from build123d import *

# Parameters (mm, degrees)
SKETCH1_W                      = 347.1920001
SKETCH1_H                      = 182.714000078
BASE_FLANGE1_DEPTH             = 2.286
EDGE_FLANGE1_STRIP_W           = 10.7696
EDGE_FLANGE1_STRIP_H           = 2.286
EDGE_FLANGE1_STRIP_CUT_DEPTH   = 182.714000078
EDGE_FLANGE1_STRIP_2_W         = 10.7696
EDGE_FLANGE1_STRIP_2_H         = 2.286
EDGE_FLANGE1_STRIP_CUT_2_DEPTH = 182.714000078
EDGE_FLANGE1_DEPTH             = 182.714000078
EDGE_FLANGE1_BEND_DEPTH        = 182.714000078
EDGE_FLANGE2_STRIP_W           = 10.7696
EDGE_FLANGE2_STRIP_H           = 2.286
EDGE_FLANGE2_STRIP_CUT_DEPTH   = 345.5664001
EDGE_FLANGE2_DEPTH             = 345.5664001
SKETCH17_W                     = 40
SKETCH17_H                     = 31.75
CUT_EXTRUDE1_DEPTH             = 201.869732409
FILLET1_R                      = 2.54
F_1_8_0_1250_DOWEL_HOLE1_D     = 3.175
F_1_8_0_1250_DOWEL_HOLE1_DEPTH = 351.7640001
F_1_8_0_1250_DOWEL_HOLE1_TIP   = 0.953866233


# Sheet-metal steps are written as plain solids
with BuildPart() as part:
    # Sketch1 → Base-Flange1 (new body)
    with BuildSketch(Plane.XY):
        Rectangle(SKETCH1_W, SKETCH1_H)
    extrude(amount=-BASE_FLANGE1_DEPTH)

    # Edge-Flange1 strip (across the edge) → Edge-Flange1 strip cut (cut)
    with BuildSketch(Plane(origin=(173.59600005, 91.357000039, -2.286), x_dir=(-1, 0, 0), z_dir=(0, -1, 0))):
        with Locations((-4.572, -1.143)):
            Rectangle(EDGE_FLANGE1_STRIP_W, EDGE_FLANGE1_STRIP_H)
    extrude(amount=EDGE_FLANGE1_STRIP_CUT_DEPTH, mode=Mode.SUBTRACT)

    # Edge-Flange1 strip 2 (across the edge) → Edge-Flange1 strip cut 2 (cut)
    with BuildSketch(Plane(origin=(-173.59600005, -91.357000039, -2.286), x_dir=(1, 0, 0), z_dir=(0, 1, 0))):
        with Locations((-4.572, -1.143)):
            Rectangle(EDGE_FLANGE1_STRIP_2_W, EDGE_FLANGE1_STRIP_2_H)
    extrude(amount=EDGE_FLANGE1_STRIP_CUT_2_DEPTH, mode=Mode.SUBTRACT)

    # Edge-Flange1 section (across the edge) → Edge-Flange1 (add)
    with BuildSketch(Plane(origin=(173.59600005, 91.357000039, -2.286), x_dir=(-1, 0, 0), z_dir=(0, -1, 0))):
        with BuildLine():
            Line((-2.286, 0.8128), (-2.286, 25.4))
            Line((-2.286, 25.4), (0, 25.4))
            Line((0, 25.4), (0, 0.8128))
            ThreePointArc((0, 0.8128), (0.238063608, 0.238063608), (0.8128, 0))
            Line((0.8128, 0), (0.8128, -2.286))
            ThreePointArc((0.8128, -2.286), (-1.378382494, -1.378382494), (-2.286, 0.8128))
        make_face()
    extrude(amount=EDGE_FLANGE1_DEPTH)

    # Edge-Flange1 section 2 (across the edge) → Edge-Flange1 bend (add)
    with BuildSketch(Plane(origin=(-173.59600005, -91.357000039, -2.286), x_dir=(1, 0, 0), z_dir=(0, 1, 0))):
        with BuildLine():
            Line((-2.286, 0.8128), (-2.286, 25.4))
            Line((-2.286, 25.4), (0, 25.4))
            Line((0, 25.4), (0, 0.8128))
            ThreePointArc((0, 0.8128), (0.238063608, 0.238063608), (0.8128, 0))
            Line((0.8128, 0), (0.8128, -2.286))
            ThreePointArc((0.8128, -2.286), (-1.378382494, -1.378382494), (-2.286, 0.8128))
        make_face()
    extrude(amount=EDGE_FLANGE1_BEND_DEPTH)

    # Edge-Flange2 strip (across the edge) → Edge-Flange2 strip cut (cut)
    with BuildSketch(Plane(origin=(172.78320005, -91.357000039, -2.286), x_dir=(0, 1, 0), z_dir=(-1, 0, 0))):
        with Locations((-4.572, -1.143)):
            Rectangle(EDGE_FLANGE2_STRIP_W, EDGE_FLANGE2_STRIP_H)
    extrude(amount=EDGE_FLANGE2_STRIP_CUT_DEPTH, mode=Mode.SUBTRACT)

    # Edge-Flange2 section (across the edge) → Edge-Flange2 (add)
    with BuildSketch(Plane(origin=(172.78320005, -91.357000039, -2.286), x_dir=(0, 1, 0), z_dir=(-1, 0, 0))):
        with BuildLine():
            Line((-2.286, 0.8128), (-2.286, 19.05))
            Line((-2.286, 19.05), (0, 19.05))
            Line((0, 19.05), (0, 0.8128))
            ThreePointArc((0, 0.8128), (0.238063608, 0.238063608), (0.8128, 0))
            Line((0.8128, 0), (0.8128, -2.286))
            ThreePointArc((0.8128, -2.286), (-1.378382494, -1.378382494), (-2.286, 0.8128))
        make_face()
    extrude(amount=EDGE_FLANGE2_DEPTH)

    # Sketch17 → Cut-Extrude1 (cut, through all)
    with BuildSketch(Plane(origin=(0, 0, -2.286), x_dir=(-1, 0, 0), z_dir=(0, 0, -1))):
        with Locations((152.78320005, 75.482000039)):
            Rectangle(SKETCH17_W, SKETCH17_H)
    extrude(amount=-CUT_EXTRUDE1_DEPTH, mode=Mode.SUBTRACT)

    # Fillet1
    fillet1_edges = [part.edges().sort_by_distance(p)[0] for p in [
        (172.78320005, -92.500000039, -21.336),
        (-172.78320005, -92.500000039, -21.336),
        (-172.78320005, 59.607000039, -1.143),
        (-132.78320005, 59.607000039, -1.143),
        (-132.78320005, 91.357000039, -1.143),
        (174.73900005, 91.357000039, -27.686),
        (174.73900005, -91.357000039, -27.686),
        (-174.73900005, -91.357000039, -27.686),
        (-174.73900005, 91.357000039, -27.686),
    ]]
    fillet(fillet1_edges, radius=FILLET1_R)

    # 1/8 (0.1250) Dowel Hole1
    with Locations(Plane.ZY.offset(175.88200005)):
        with Locations((-14.1224, -72.307000039), (-14.1224, 78.657000039)):
            Hole(F_1_8_0_1250_DOWEL_HOLE1_D / 2, depth=F_1_8_0_1250_DOWEL_HOLE1_DEPTH)
            with Locations((0, 0, -(F_1_8_0_1250_DOWEL_HOLE1_DEPTH + F_1_8_0_1250_DOWEL_HOLE1_TIP / 2))):  # 118° drill point
                Cone(0, F_1_8_0_1250_DOWEL_HOLE1_D / 2, F_1_8_0_1250_DOWEL_HOLE1_TIP, mode=Mode.SUBTRACT)


solid = part.part
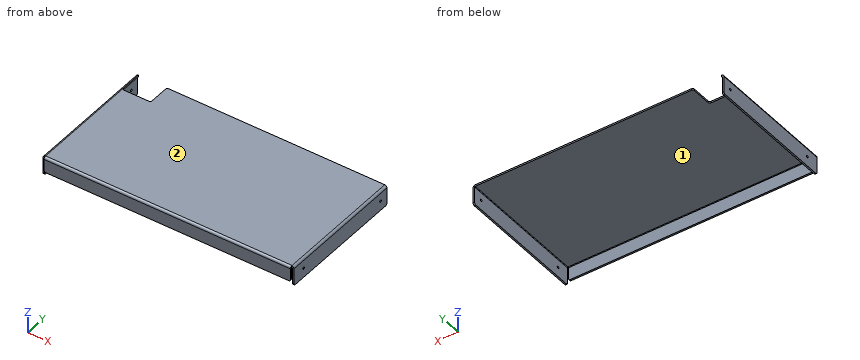
Source: CAD feature listing. Evaluate the final solid. Frame: model axes, mm. Face numbers are marked on the shaded views. Round coordinates to 2 decimals unless told otherwise and drop trailing zeros. Loops run counter-clockwise (first coordinate to the right, second up) from the corner with the lowest first, then second, coordinate; pieces in that order, holes last. Notation, with made-up numbers: M 63,54.25 L 105,54.25 A32 ccw 105,84.25 Z; hole C 69,-38 d1. An arc over 180 degrees is marked long. Return JSON: item names as keys, results as strings. Group by question number.
1. Section query D-D on y = -4. Output: boundary loops of the cut face in (x, z), and give its area (3 significant figures).
2. Section query A-A on y = 68. Output: boundary loops of the cut face in (x, z), and give its area (3 significant figures).
3. Material intervals for line 1 along X through (y, z) = (51, -10); line 2 along Y through (x, z) = (92, -21.25); line 3 along Z through (x, y) = (135, -30), sorted ascending. Write a range as from..to.
4. Pin query (flat end, axial travel): pin 1 (1.8 mm diameter, centred on y = 70, z = -1.5, fed in from -X); pin 2 (4 mm diameter, centred on y = 78.66, z = -14.12, fed in from +X); pin 3 (10 mm diameter, centred on x = -110, z = -16, fed in from +Y); pin 4 (6 mm diameter, centred on x = -44.5, y = -46.5, fed in from -Z). Return the tip coordinate at first contact, or that it passes through.
5. Section query C-C on x = -28.5. Output: boundary loops of the cut face in (y, z), and give its area (3 significant figures).
6. Section query B-B on z = -9. Output: boundary loops of the cut face in (x, y), and give its area (3 significant figures).
7. Mould query, pull axis X, two halves, no side actions, for the marked faces 1 and 2. Classes: released by +X, released by -X, zero draft, split by the parting line, or undercut.
Checks:
{
 "1": {"outline": "M -175.88,-27.69 L -173.6,-27.69 L -173.6,-3.1 A0.81 cw -172.78,-2.29 L 172.78,-2.29 A0.81 cw 173.6,-3.1 L 173.6,-27.69 L 175.88,-27.69 L 175.88,-3.1 A3.1 ccw 172.78,0 L -172.78,0 A3.1 ccw -175.88,-3.1 Z", "area": "916 mm²"},
 "2": {"outline": "M -175.88,-27.69 L -173.6,-27.69 L -173.6,-3.1 A0.81 cw -172.78,-2.29 L -172.78,0 A3.1 ccw -175.88,-3.1 Z; M -132.78,-2.29 L 172.78,-2.29 A0.81 cw 173.6,-3.1 L 173.6,-27.69 L 175.88,-27.69 L 175.88,-3.1 A3.1 ccw 172.78,0 L -132.78,0 Z", "area": "825 mm²"},
 "3": {"line 1": "x = -175.88..-173.6, 173.6..175.88", "line 2": "y = -93.64..-91.36", "line 3": "z = -2.29..0"},
 "4": {"pin 1": "stops at x = -175.8", "pin 2": "stops at x = 175.88", "pin 3": "stops at y = -91.36", "pin 4": "stops at z = -2.29"},
 "5": {"outline": "M -93.64,-21.34 L -91.36,-21.34 L -91.36,-3.1 A0.81 cw -90.54,-2.29 L 91.36,-2.29 L 91.36,0 L -90.54,0 A3.1 ccw -93.64,-3.1 Z", "area": "465 mm²"},
 "6": {"outline": "M -175.88,-91.36 L -173.6,-91.36 L -173.6,91.36 L -175.88,91.36 Z; M -172.78,-93.64 L 172.78,-93.64 L 172.78,-91.36 L -172.78,-91.36 Z; M 173.6,-91.36 L 175.88,-91.36 L 175.88,91.36 L 173.6,91.36 Z", "area": "1,630 mm²"},
 "7": {"face 1": "undercut", "face 2": "zero draft"}
}
